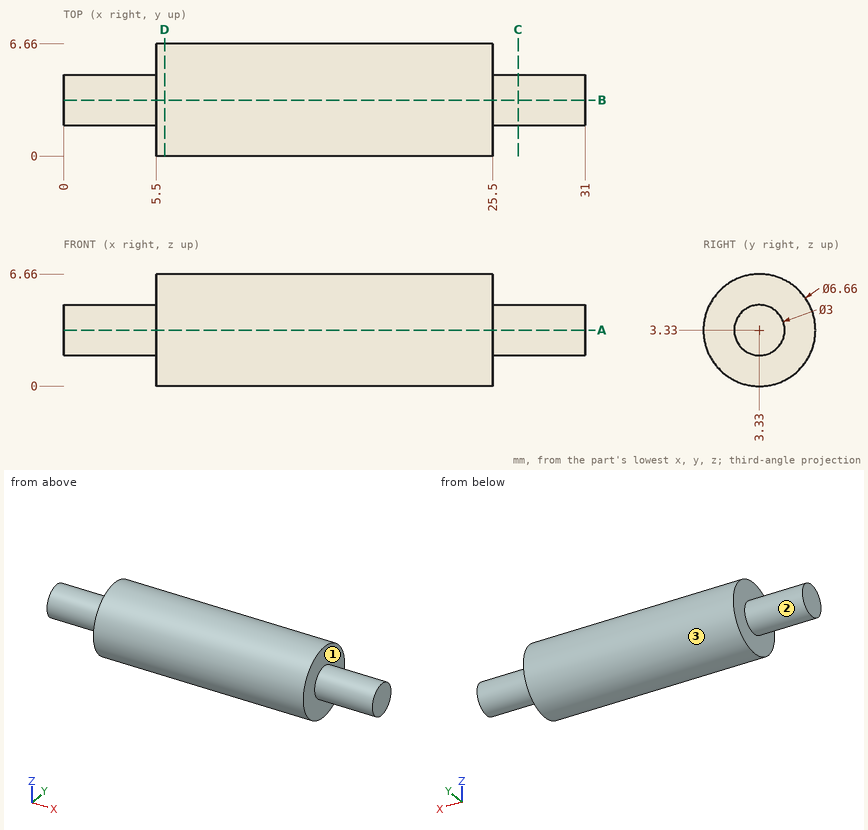
The drawing under review shows one solid part. Ordinate dimensions are in mm from its lowest x, y, z. A direction names the side the tool comes from. Give positions to 0.01 mm unless a question says otherwise; leave off trailing zeros. Order: outer loops, then holes, each group sorted by start corner. A loop starts at its lowest first (then second) coordinate and runs counter-clockwise, first axis right, second up. Notation, with made-up numbers: M -30,82.25 L 26,82.25 A15 ccw 26,86.25 Z; hole C 16,9.25 d3. An arc over 180 degrees is marked long. One line per question, with ' | ' between items. Start each with the question number.
Q1. For L1, parallel to X at y = 5.5, z = 4; L2, parallel to Y at x = 4.5, z = 3.5; L3, parallel to Y at x = 14, z = 3, list the stretches that pass through material, from the lowest coordinate up. Write a range as [from, to].
Q2. Machinability: for the marked faces 1, 2 and 3, which of the approach directions +Z, -Z, +X, -X, +Y, -Y give a long, thin tool a straight path to every point of the face, cutting with its end or side? Answer none if there is none.
Q3. We need section C-C (x = 27). Write out the cut boundary in (y, z), plus the area to 3 significant figures.
Q4. We need section A-A (z = 3.33). Write out the cut boundary in (x, y).
Q5. We need section D-D (x = 6). Write out the cut boundary in (y, z).
Q6. For pin 1 Ø1 at (y, z) = (2, 1) entering from +X; pin 2 Ø3 at (x, y) = (3.5, 4) entering from +Z, all flat-tipped, find the tip position at first contact; note any pin that passes through.
Returned:
1) L1: [5.5, 25.5] | L2: [1.84, 4.82] | L3: [0.02, 6.64]
2) face 1: +X | face 2: -X | face 3: +X, -X
3) outline: C 3.33,3.33 d3 | area: 7.07 mm2
4) outline: M 0,1.83 L 5.5,1.83 L 5.5,0 L 25.5,0 L 25.5,1.83 L 31,1.83 L 31,4.83 L 25.5,4.83 L 25.5,6.66 L 5.5,6.66 L 5.5,4.83 L 0,4.83 Z
5) outline: C 3.33,3.33 d6.66
6) pin 1: x = 25.5 | pin 2: z = 4.83
